Geometry: final body of the model. Coordinates: model frame, mm. A direction names the side the tool comes from. Coordinates: 2 decimals unless noted, no trailing zeros. Order: outer loops, then holes, each group sorted by start corner. A loop starts at its lowest first (then second) coordinate and runs counter-clockwise, first axis right, second up. Notation, with made-up numbers: M 63,87 L 74,87 A23 ccw 74,111 Z; hole C 61,-2 d7. An arc over 180 degrees is marked long. One line per question, with ' | ' between items.
from build123d import *

# Parameters (mm, degrees)
SIDES_DEPTH           = 8
SKETCH2_W             = 5
SKETCH2_H             = 4
FRONT_CUT_DEPTH       = 0.5
BACK_CUT_REACH        = 15.748
SKETCH3_W             = 5
SKETCH3_H             = 1
BASE_DEPTH            = 0.5
PINS_DEPTH            = 4
PINS_DEPTH_BACK       = 3.5
SKETCH4_W             = 0.635
SKETCH4_H             = 0.635
CLIP_DEPTH            = 2
CLIP_DEPTH_BACK       = 2
FRONT_TRIM_DEPTH      = 11.677078252
FRONT_TRIM_DEPTH_BACK = 11.677078252
SKETCH6_W             = 0.5
SKETCH6_H             = 1.5
BOSS_EXTRUDE4_DEPTH   = 1.51


with BuildPart() as part:
    # Sketch1 → Sides (new body)
    with BuildSketch(Plane(origin=(0, 0, 0), x_dir=(1, 0, 0), z_dir=(0, 1, 0))):
        Polygon((8.5, 0), (10, 0), (10, 5), (0, 5), (0, 0), (1.5, 0), (1.5, 0.5), (8.5, 0.5), align=None)
        Polygon((0.5, 4.5), (9.5, 4.5), (9.5, 1.528846154), (9.5, 0.5), (9, 0.5), (9, 1), (1, 1), (1, 0.5), (0.5, 0.5), (0.5, 1.538461538), align=None, mode=Mode.SUBTRACT)
    extrude(amount=SIDES_DEPTH)

    # Sketch2 → Front cut (cut)
    with BuildSketch(Plane.XY.offset(-0.5)):
        with Locations((5, 6)):
            Rectangle(SKETCH2_W, SKETCH2_H)
    extrude(amount=-FRONT_CUT_DEPTH, mode=Mode.SUBTRACT)

    # Sketch3 → Back cut (cut, up to next)
    with BuildSketch(Plane(origin=(0, 0, -5), x_dir=(-1, 0, 0), z_dir=(0, 0, -1)), mode=Mode.PRIVATE) as back_cut_sk1:
        with Locations((-5, 7.5)):
            Rectangle(SKETCH3_W, SKETCH3_H)
    back_cut_tool1 = extrude(back_cut_sk1.sketch, amount=-BACK_CUT_REACH, mode=Mode.PRIVATE) & part.part
    add(back_cut_tool1.solids().sort_by_distance((5, 7.5, -5))[0], mode=Mode.SUBTRACT)

    # Sketch1<2> → Base (add)
    with BuildSketch(Plane(origin=(0, 0, 0), x_dir=(1, 0, 0), z_dir=(0, 1, 0))):
        Polygon((1, 1), (1, 0.5), (0.5, 0.5), (0.5, 1.538461538), (0.5, 4.5), (9.5, 4.5), (9.5, 1.528846154), (9.5, 0.5), (9, 0.5), (9, 1), align=None)
    extrude(amount=BASE_DEPTH)

    # Sketch4 → Pins (add, two sides: drawn at the far end of the back side and taken through both)
    with BuildSketch(Plane(origin=(0, 0.5, 0), x_dir=(1, 0, 0), z_dir=(0, 1, 0)).offset(-PINS_DEPTH_BACK)):
        with Locations((2, 2.5)):
            Rectangle(SKETCH4_W, SKETCH4_H)
        with Locations((4, 2.5)):
            Rectangle(SKETCH4_W, SKETCH4_H)
        with Locations((6, 2.5)):
            Rectangle(SKETCH4_W, SKETCH4_H)
        with Locations((8, 2.5)):
            Rectangle(SKETCH4_W, SKETCH4_H)
    extrude(amount=PINS_DEPTH + PINS_DEPTH_BACK)

    # Sketch5 → Clip (add, two sides: drawn at the far end of the back side and taken through both)
    with BuildSketch(Plane(origin=(5, 0, 0), x_dir=(0, 0, -1), z_dir=(1, 0, 0)).offset(-CLIP_DEPTH_BACK)):
        Polygon((0.5, 4), (0.5, 3), (0, 2.8), (0, 3.3), align=None)
    extrude(amount=CLIP_DEPTH + CLIP_DEPTH_BACK)

    # Sketch6 → Front trim (cut, two sides: drawn at the far end of the back side and taken through both)
    with BuildSketch(Plane(origin=(5, 0, 0), x_dir=(0, 0, -1), z_dir=(1, 0, 0)).offset(-FRONT_TRIM_DEPTH_BACK)):
        with Locations((0.25, 0.75)):
            Rectangle(SKETCH6_W, SKETCH6_H)
    extrude(amount=FRONT_TRIM_DEPTH + FRONT_TRIM_DEPTH_BACK, mode=Mode.SUBTRACT)

    # Sketch1<4> → Boss-Extrude4 (add)
    with BuildSketch(Plane(origin=(0, 0, 0), x_dir=(1, 0, 0), z_dir=(0, 1, 0))):
        Polygon((1, 1), (1, 0.5), (0.5, 0.5), (0.5, 1.538461538), (0.5, 4.5), (9.5, 4.5), (9.5, 1.528846154), (9.5, 0.5), (9, 0.5), (9, 1), align=None)
    extrude(amount=BOSS_EXTRUDE4_DEPTH)


solid = part.part
1. Section B-B, the plane y = -1. Output: boundary loops of the cut face in (x, z), and give its area (3 significant figures).
Response values:
outline: M 1.68,-2.82 L 2.32,-2.82 L 2.32,-2.18 L 1.68,-2.18 Z; M 3.68,-2.82 L 4.32,-2.82 L 4.32,-2.18 L 3.68,-2.18 Z; M 5.68,-2.82 L 6.32,-2.82 L 6.32,-2.18 L 5.68,-2.18 Z; M 7.68,-2.82 L 8.32,-2.82 L 8.32,-2.18 L 7.68,-2.18 Z | area: 1.61 mm^2
2. Pin query (flat end, axial travel): P1, Ø3, axis at x = 2, z = -1.5, coming from the -Y side. Return the tip coordinate at first contact, or that it passes through.
Response values:
P1: stops at y = -3
3. Section A-A, the plane y = 7.25. Output: boundary loops of the cut face in (x, z), and give its area (3 significant figures).
Response values:
outline: M 0,-5 L 2.5,-5 L 2.5,-4.5 L 0.5,-4.5 L 0.5,-0.5 L 1,-0.5 L 1,-1 L 2.5,-1 L 2.5,-0.5 L 1.5,-0.5 L 1.5,0 L 0,0 Z; M 7.5,-5 L 10,-5 L 10,0 L 8.5,0 L 8.5,-0.5 L 7.5,-0.5 L 7.5,-1 L 9,-1 L 9,-0.5 L 9.5,-0.5 L 9.5,-4.5 L 7.5,-4.5 Z | area: 9.50 mm^2
4. Section D-D, the plane z = -0.85. Output: boundary loops of the cut face in (x, y).
Response values:
outline: M 0,0 L 10,0 L 10,8 L 9.5,8 L 9.5,1.51 L 9,1.51 L 9,8 L 7.5,8 L 7.5,4 L 2.5,4 L 2.5,8 L 1,8 L 1,1.51 L 0.5,1.51 L 0.5,8 L 0,8 Z
5. Section C-C, the plane x = 7.25. Output: boundary loops of the cut face in (y, z).
Response values:
outline: M 0,-5 L 7,-5 L 7,-4.5 L 1.51,-4.5 L 1.51,-1 L 4,-1 L 4,-0.5 L 0,-0.5 Z
6. Material intervals for line 1 (Z direction, x = 9.25, y = 7.5); line 2 (X direction, y = 5.25, z = -3.05); line 3 (X direction, y = -0.25, z = -2.7), sorted ascending. Write a range as [from, to].
Response values:
line 1: z = [-5, -4.5], [-0.5, 0] | line 2: x = [0, 0.5], [9.5, 10] | line 3: x = [1.68, 2.32], [3.68, 4.32], [5.68, 6.32], [7.68, 8.32]
7. Access query for faces 4 (the face through (9, 5, 0)), 5 (the face through (5, 3, -1)). Directions: +Z, -Z, +X, -X, +Y, -Y. A direction counts if a zero-diameter tool reaches every point of the face in a straight line with its end or side. Return the directions, or none.
Response values:
face 4: +Z, +X, -X, +Y, -Y | face 5: +Y
8. Draft query along Z for faces 1 (the face through (9.5, 5, -3)), 2 (the face through (9.8, 8, -2.5)), 3 (the face through (1, 5, 0)). Return one class per face: pulls with the +Z half, pulls with the -Z half, needs draft (parallel to the pull), parting line crosses it, or undercut.
Response values:
face 1: undercut | face 2: needs draft | face 3: pulls with the +Z half
